```python
from build123d import *

# Parameters (mm, degrees)
SKETCH1_R           = 3.175
BOSS_EXTRUDE1_DEPTH = 137.2
BOSS_EXTRUDE2_START = -15.88
SKETCH2_R           = 4.7625
BOSS_EXTRUDE2_DEPTH = 105.45
CUT_EXTRUDE1_START  = 9.53
SKETCH4_R           = 3.175
SKETCH4_R_2         = 2.665
CUT_EXTRUDE1_DEPTH  = 2


with BuildPart() as part:
    # Sketch1 → Boss-Extrude1 (new body)
    with BuildSketch(Plane(origin=(0, 0, 0), x_dir=(1, 0, 0), z_dir=(0, 1, 0))):
        with Locations(Location((0, 0, 0), (0, 0, 270))):
            Circle(SKETCH1_R)
    extrude(amount=BOSS_EXTRUDE1_DEPTH)

    # Sketch2 → Boss-Extrude2 (add)
    with BuildSketch(Plane(origin=(0, 137.2, 0), x_dir=(1, 0, 0), z_dir=(0, 1, 0)).offset(BOSS_EXTRUDE2_START)):
        with Locations(Location((0, 0, 0), (0, 0, 270))):
            Circle(SKETCH2_R)
    extrude(amount=-BOSS_EXTRUDE2_DEPTH)

    # Sketch4 → Cut-Extrude1 (cut)
    with BuildSketch(Plane(origin=(0, 121.32, 0), x_dir=(1, 0, 0), z_dir=(0, 1, 0)).offset(CUT_EXTRUDE1_START)):
        with Locations(Location((0, 0, 0), (0, 0, 270))):
            Circle(SKETCH4_R)
        with Locations(Location((0, 0, 0), (0, 0, 270))):
            Circle(SKETCH4_R_2, mode=Mode.SUBTRACT)
    cut_extrude1 = extrude(amount=CUT_EXTRUDE1_DEPTH, mode=Mode.SUBTRACT)

    # Mirror1: Cut-Extrude1 across plane
    add(cut_extrude1.mirror(Plane.ZX.offset(68.595)), mode=Mode.SUBTRACT)


solid = part.part
```
Geometry check sheet. Reference: the model listing, model coordinates, mm. A direction names the side the tool comes from. Coordinates: 2 decimals unless noted, no trailing zeros. Order: outer loops, then holes, each group sorted by start corner. A loop starts at its lowest first (then second) coordinate and runs counter-clockwise, first axis right, second up.
Q1. Tool access check on faces 5 (the face through (-2.9, 69.33, -3.78)), 6 (the face through (-1.93, 134.99, -2.52)), 7 (the face through (-2.6, 131.84, -0.58)), 8 (the face through (-1.93, 2.14, -2.52)). Record the directions out of +Z, -Z, +X, -X, +Y, -Y that give a thin tool (end or side, any length) a straight path to the whole face; none if there is none.
Reply:
face 5: +Y, -Y
face 6: +Y
face 7: none
face 8: -Y
Q2. Draft check along Y on faces 1 (the face through (-2.6, 5.35, -0.58)), 2 (the face through (-1.93, 126.02, -2.52)), 3 (the face through (0, 137.2, 0)), 4 (the face through (0, 0, 0)). Enter one of: released by +Y, released by -Y, zero draft, split by the parting line, or undercut.
Reply:
face 1: undercut
face 2: zero draft
face 3: released by +Y
face 4: released by -Y
Q3. Thickness scan on probe 1 along Y at (x, z) = (1.5, -2.75); probe 2 along X at (y, z) = (22, -0.5); probe 3 along X at (y, z) = (128, -1.75). Record the ranges inside material, lowest first.
Reply:
probe 1: y = 0 to 4.34, 6.34 to 130.85, 132.85 to 137.2
probe 2: x = -4.74 to 4.74
probe 3: x = -2.65 to 2.65
Q4. Depth check by flat-ended pin: pin 1 Ø1 at (x, z) = (0.5, -4) entering from -Y; pin 2 Ø5 at (x, y) = (-3, 21.5) entering from +Z; pin 3 Ø2 at (y, z) = (108, 3.5) entering from +X. Enter the tip coordinate at first touch or a pass-through.
Reply:
pin 1: stops at y = 15.87
pin 2: stops at z = 4.74
pin 3: stops at x = 4.05
Q5. Sectioned sample at B-B on y = 44. Record the cut outline in (x, z) (1 decimal), and give its area (3 significant figures).
Reply:
outline: circle Ø9.5 at (0, 0)
area: 71.3 mm2
